```python
from build123d import *

# Parameters (mm, degrees)
F1_DEPTH = 2
F3_DEPTH = 1
F4_R     = 1


with BuildPart() as f1:
    # F0 (on Top) → F1 (new body)
    with BuildSketch(Plane.XY):
        with BuildLine():
            ThreePointArc((4.298409, 1.1516), (4.426787, -0.453934), (3.975236, -2))
            Line((3.975236, -2), (23.632209, 17.656973))
            ThreePointArc((23.632209, 17.656973), (0, 29.5), (-23.632209, 17.656973))
            Line((-23.632209, 17.656973), (-3.975236, -2))
            ThreePointArc((-3.975236, -2), (-4.426787, -0.453934), (-4.298409, 1.1516))
            Line((-4.298409, 1.1516), (-20.955081, 17.808273))
            ThreePointArc((-20.955081, 17.808273), (0, 27.5), (20.955081, 17.808273))
            Line((20.955081, 17.808273), (4.298409, 1.1516))
        make_face()
        with BuildLine():
            Line((0.5, -3.413576), (0.5, -4.421821))
            ThreePointArc((0.5, -4.421821), (2.544256, -3.650926), (3.975236, -2))
            ThreePointArc((3.975236, -2), (4.426787, -0.453934), (4.298409, 1.1516))
            ThreePointArc((4.298409, 1.1516), (0, 4.45), (-4.298409, 1.1516))
            ThreePointArc((-4.298409, 1.1516), (-4.426787, -0.453934), (-3.975236, -2))
            ThreePointArc((-3.975236, -2), (-2.544256, -3.650926), (-0.5, -4.421821))
            Line((-0.5, -4.421821), (-0.5, -3.413576))
            ThreePointArc((-0.5, -3.413576), (0, 3.45), (0.5, -3.413576))
        make_face()
    extrude(amount=F1_DEPTH)

    # F2 (on face) → F3 (join)
    with BuildSketch(Plane.XY.offset(2)):
        with BuildLine():
            Line((0.45, 3.420526), (0.45, 4.427189))
            ThreePointArc((0.45, 4.427189), (0, 4.45), (-0.45, 4.427189))
            Line((-0.45, 4.427189), (-0.45, 3.420526))
            ThreePointArc((-0.45, 3.420526), (0, 3.45), (0.45, 3.420526))
        make_face()
    extrude(amount=F3_DEPTH)

    # F4
    f4_edges = [f1.edges().sort_by_distance(p)[0] for p in [
        (-23.632209, 17.656973, 1),
        (-20.955081, 17.808273, 1),
        (23.632209, 17.656973, 1),
        (20.955081, 17.808273, 1),
    ]]
    fillet(f4_edges, radius=F4_R)


solid = f1.part
```
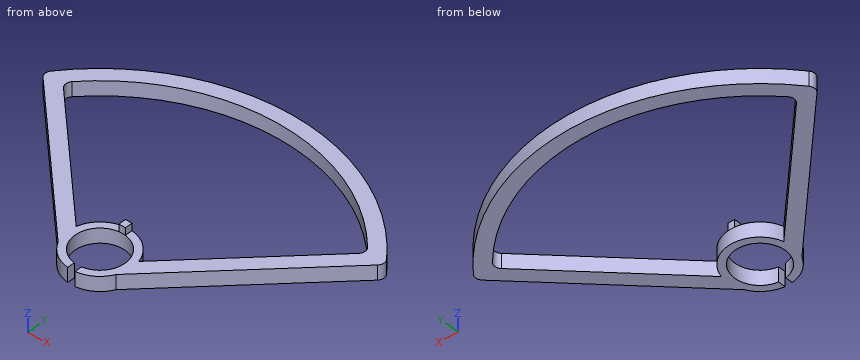
Geometry: final body of the model. Coordinates: model frame, mm. Give positions to 0.01 mm unless a question says otherwise; leave off trailing zeros. Order: outer loops, then holes, each group sorted by start corner. A loop starts at its lowest first (then second) coordinate and runs counter-clockwise, first axis right, second up. Notation, with made-up numbers: (39.25, -30) -> (65.25, -30) arc R31 ccw to (65.25, -2) -> close; hole circle Ø5 at (-5, -19.75). An arc over 180 degrees is marked (long way). Write each question's results on one line, items separated by ' | '. Start each with the question number.
1) Line query: line 1 (Y direction, x = 0, z = 1.3); line 2 (X direction, y = 1.5, z = 1.1); line 3 (Y direction, x = 1, z = 1.3). Output: solid intervals per line, ascending. Write a range as from..to.
2) Section D-D (y = 2). Return loops of the section in (x, z), then the cut area to 3 significant figures.
3) Section B-B (z = 1.5). Return loops of the section in (x, y), then the cut area to 3 significant figures.
4) Section C-C (y = 11). Return loops of the section in (x, z), then the cut area to 3 significant figures.
5) First-contact query: pin 1 (1.5 mm diameter, centred on y = 7.5, z = 1.5, fed in from -X); pin 2 (1.5 mm diameter, centred on y = 15.5, z = 2, fed in from -X); pin 3 (2 mm diameter, centred on x = -2.5, y = 2.5, fed in from -Z); pin 4 (0.5 mm diameter, centred on y = 3.5, z = 2.5, fed in from -X). Flat tips, straight axial feed; report the tip coordinate or a pass-through.
6) Section A-A (x = -2). Return loops of the section in (y, z), then the cut area to 3 significant figures.
Calculated:
1) line 1: 3.45..4.45, 27.5..29.5 | line 2: -7.48..-4.65, -4.19..-3.11, 3.11..4.19, 4.65..7.48 | line 3: -4.34..-3.3, 3.3..4.34, 27.48..29.48
2) outline: (-7.98, 0) -> (-5.15, 0) -> (-5.15, 2) -> (-7.98, 2) -> close; (-3.98, 0) -> (-2.81, 0) -> (-2.81, 2) -> (-3.98, 2) -> close; (2.81, 0) -> (3.98, 0) -> (3.98, 2) -> (2.81, 2) -> close; (5.15, 0) -> (7.98, 0) -> (7.98, 2) -> (5.15, 2) -> close | area: 16.0 mm2
3) outline: (-23.09, 18.37) arc R1 ccw to (-23.01, 17.04) -> (-3.98, -2) arc R4.45 ccw to (-0.5, -4.42) -> (-0.5, -3.41) arc R3.45 cw (long way) to (0.5, -3.41) -> (0.5, -4.42) arc R4.45 ccw to (3.98, -2) -> (23.01, 17.04) arc R1 ccw to (23.09, 18.37) arc R29.5 ccw to start; hole (-20.32, 18.53) arc R1 ccw to (-20.29, 17.14) -> (-4.3, 1.15) arc R4.45 cw to (4.3, 1.15) -> (20.29, 17.14) arc R1 ccw to (20.32, 18.53) arc R27.5 ccw to start | area: 228 mm2
4) outline: (-16.98, 0) -> (-14.15, 0) -> (-14.15, 2) -> (-16.98, 2) -> close; (14.15, 0) -> (16.98, 0) -> (16.98, 2) -> (14.15, 2) -> close | area: 11.3 mm2
5) pin 1: x = -14.23 | pin 2: x = -22.23 | pin 3: z = 0 | pin 4: x = -0.45
6) outline: (-3.98, 0) -> (-2.81, 0) -> (-2.81, 2) -> (-3.98, 2) -> close; (2.81, 0) -> (3.98, 0) -> (3.98, 2) -> (2.81, 2) -> close; (27.43, 0) -> (29.43, 0) -> (29.43, 2) -> (27.43, 2) -> close | area: 8.67 mm2
